```python
from build123d import *

# Parameters (mm, degrees)
ESBO_O1_W                = 156.68
ESBO_O1_H                = 216
ESBO_O1_W_2              = 67.84
ESBO_O1_H_2              = 97.5
RESSALTO_EXTRUS_O1_DEPTH = 3
ESBO_O2_R                = 3
RESSALTO_EXTRUS_O2_DEPTH = 3
ESBO_O3_R                = 2
CORTE_EXTRUS_O1_DEPTH    = 1


with BuildPart() as part:
    # Esboço1 → Ressalto-extrusão1 (new body)
    with BuildSketch(Plane.XY):
        Rectangle(ESBO_O1_W, ESBO_O1_H)
        with Locations((-37.42, 52.25)):
            Rectangle(ESBO_O1_W_2, ESBO_O1_H_2, mode=Mode.SUBTRACT)
        with Locations((37.42, 52.25)):
            Rectangle(ESBO_O1_W_2, ESBO_O1_H_2, mode=Mode.SUBTRACT)
        with Locations((-37.42, -52.25)):
            Rectangle(ESBO_O1_W_2, ESBO_O1_H_2, mode=Mode.SUBTRACT)
        with Locations((37.42, -52.25)):
            Rectangle(ESBO_O1_W_2, ESBO_O1_H_2, mode=Mode.SUBTRACT)
    extrude(amount=RESSALTO_EXTRUS_O1_DEPTH)

    # Esboço2 → Ressalto-extrusão2 (add)
    with BuildSketch(Plane.XY.offset(3)):
        Circle(ESBO_O2_R)
    extrude(amount=RESSALTO_EXTRUS_O2_DEPTH)

    # Esboço3 → Corte-extrusão1 (cut)
    with BuildSketch(Plane(origin=(0, 0, 0), x_dir=(-1, 0, 0), z_dir=(0, 0, -1))):
        with Locations((-74.34, 104)):
            Circle(ESBO_O3_R)
        with Locations((74.34, 104)):
            Circle(ESBO_O3_R)
        with Locations((74.34, -104)):
            Circle(ESBO_O3_R)
        with Locations((-74.34, -104)):
            Circle(ESBO_O3_R)
    extrude(amount=-CORTE_EXTRUS_O1_DEPTH, mode=Mode.SUBTRACT)


solid = part.part
```
CAD build for the part. Positions are in the model's coordinates, mm. Coordinates: 2 decimals unless noted, no trailing zeros. Order: outer loops, then holes, each group sorted by start corner. A loop starts at its lowest first (then second) coordinate and runs counter-clockwise, first axis right, second up. Notation, with made-up numbers: (20.5, 59) - (67.5, 59) arc R11 ccw to (67.5, 80) - close; hole circle Ø2 at (84, -5). An arc over 180 degrees is marked (long way). Use a Markdown table: item, result. Add a question column.
(1) Saw through at B-B (z = 2.05). Give the cut face in (x, y), then the cut area to 3 significant figures.
(2) Saw through at C-C (x = 35). Give the cut face in (y, z), then the cut area to 3 significant figures.
(3) Saw through at D-D (x = 0). Give the cut face in (y, z).
(4) Pull direction Z, two halves, no side cores. Call faces 1 (the face through (0, 1, 0)), 2 (the face through (-3, 0, 4)), 3 (the face through (0, 0, 6)): +Z half, -Z half, draft (parallel to the pull), parting line (faces both ways), or undercut.
(5) Saw through at A-A (y = 12.5). Give the cut face in (x, z).
(6) Drill centre lines: line 1 along Y through (x, z) = (74.34, 0.55); line 2 along X through (y, z) = (-54, 1.15); line 3 along Y through (x, z) = (60.5, 2.2). Where is each one in solid material? Low to high. Write a range as [from, to].
(7) Flat gauge pins, fed straight in: pin 1 (4.5 mm diameter, centred on x = 74.34, y = -104, fed in from +Z); pin 2 (2 mm diameter, centred on x = 74, y = -103.5, fed in from -Z); pin 3 (1.5 mm diameter, centred on y = -6, z = 4, fed in from -X). Where does each tip first touch, or does it go through?
Solved:
| question | item | result |
|---|---|---|
| 1 | outline | (-78.34, -108) - (78.34, -108) - (78.34, 108) - (-78.34, 108) - close; hole (-71.34, -101) - (-3.5, -101) - (-3.5, -3.5) - (-71.34, -3.5) - close; hole (-71.34, 3.5) - (-3.5, 3.5) - (-3.5, 101) - (-71.34, 101) - close; hole (3.5, -101) - (71.34, -101) - (71.34, -3.5) - (3.5, -3.5) - close; hole (3.5, 3.5) - (71.34, 3.5) - (71.34, 101) - (3.5, 101) - close |
| 1 | area | 7,390 mm² |
| 2 | outline | (-108, 0) - (-101, 0) - (-101, 3) - (-108, 3) - close; (-3.5, 0) - (3.5, 0) - (3.5, 3) - (-3.5, 3) - close; (101, 0) - (108, 0) - (108, 3) - (101, 3) - close |
| 2 | area | 63.0 mm² |
| 3 | outline | (-108, 0) - (108, 0) - (108, 3) - (3, 3) - (3, 6) - (-3, 6) - (-3, 3) - (-108, 3) - close |
| 4 | face 1 | -Z half |
| 4 | face 2 | draft |
| 4 | face 3 | +Z half |
| 5 | outline | (-78.34, 0) - (-71.34, 0) - (-71.34, 3) - (-78.34, 3) - close; (-3.5, 0) - (3.5, 0) - (3.5, 3) - (-3.5, 3) - close; (71.34, 0) - (78.34, 0) - (78.34, 3) - (71.34, 3) - close |
| 6 | line 1 | y = [-108, -106], [-102, 102], [106, 108] |
| 6 | line 2 | x = [-78.34, -71.34], [-3.5, 3.5], [71.34, 78.34] |
| 6 | line 3 | y = [-108, -101], [-3.5, 3.5], [101, 108] |
| 7 | pin 1 | stops at z = 3 |
| 7 | pin 2 | stops at z = 1 |
| 7 | pin 3 | passes through |
